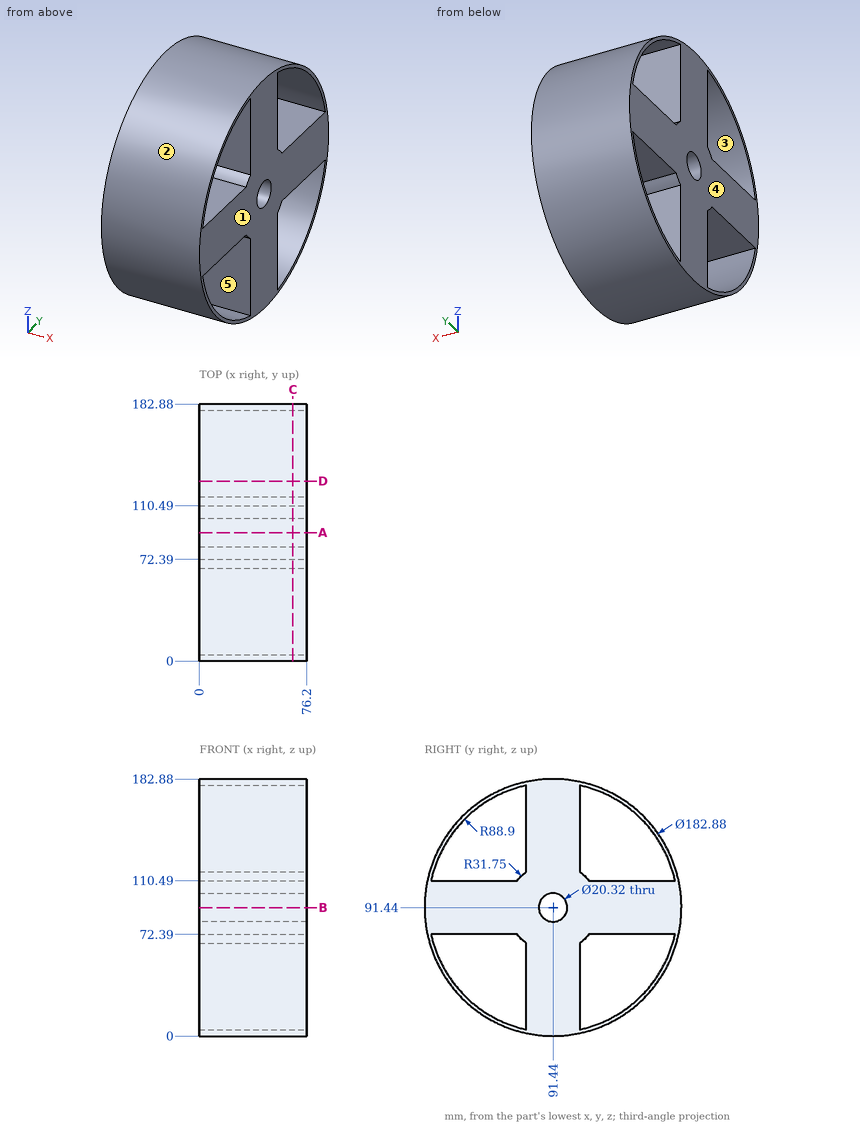
Drawing for the job (mm, zero at the part's lowest x, y, z). A direction names the side the tool comes from. Round coordinates to 2 decimals unless told otherwise and drop trailing zeros. Loops run counter-clockwise (first coordinate to the right, second up) from the corner with the lowest first, then second, coordinate; pieces in that order, holes last. Notation, with made-up numbers: (23, -28) -> (34, -28) arc R18 cw to (34, -18) -> close; hole circle Ø10 at (56.25, -13). An arc over 180 degrees is marked (long way). Answer in a Markdown table with one row per item.
Item 1: Mould opens along Z. For the marked faces 1, 2 and 3 say: +Z half, -Z half, draft (parallel to the pull), parting line (faces both ways), or undercut.
Answers below:
| item | result |
|---|---|
| face 1 | draft |
| face 2 | parting line |
| face 3 | undercut |
Item 2: Saw through at A-A (y = 91.44). Write the cut outline in (x, z), and give its area (3 significant figures).
Answers below:
| item | result |
|---|---|
| outline | (0, 0) -> (76.2, 0) -> (76.2, 81.28) -> (0, 81.28) -> close; (0, 101.6) -> (76.2, 101.6) -> (76.2, 182.88) -> (0, 182.88) -> close |
| area | 12,400 mm² |
Item 3: Saw through at D-D (y = 128). Write the cut outline in (x, z).
Answers below:
| item | result |
|---|---|
| outline | (0, 7.63) -> (76.2, 7.63) -> (76.2, 10.41) -> (0, 10.41) -> close; (0, 72.39) -> (76.2, 72.39) -> (76.2, 110.49) -> (0, 110.49) -> close; (0, 172.47) -> (76.2, 172.47) -> (76.2, 175.25) -> (0, 175.25) -> close |
Item 4: Which spindle directions (+Z, -Z, +X, -X, +Y, -Y) get a long thin tool onto all of the face, cutting with end or side? Do the marked faces 4 and 5. Say none if no direction does.
Answers below:
| item | result |
|---|---|
| face 4 | +Z, -Z, -X, +Y, -Y |
| face 5 | +X, -X |
Item 5: Saw through at C-C (x = 66.5). Write the cut outline in (y, z).
Answers below:
| item | result |
|---|---|
| outline | circle Ø182.88 at (91.44, 91.44); hole (4.61, 72.39) arc R88.9 ccw to (72.39, 4.61) -> (72.39, 66.04) arc R31.75 cw to (66.04, 72.39) -> close; hole (4.61, 110.49) -> (66.04, 110.49) arc R31.75 cw to (72.39, 116.84) -> (72.39, 178.27) arc R88.9 ccw to start; hole circle Ø20.32 at (91.44, 91.44); hole (110.49, 4.61) arc R88.9 ccw to (178.27, 72.39) -> (116.84, 72.39) arc R31.75 cw to (110.49, 66.04) -> close; hole (110.49, 116.84) arc R31.75 cw to (116.84, 110.49) -> (178.27, 110.49) arc R88.9 ccw to (110.49, 178.27) -> close |
Item 6: Drill centre lines: L1, parallel to Y at x = 52, z = 91.44; L2, parallel to Y at x = 58.5, z = 154.5; L3, parallel to Y at x = 67, z = 163.5. Where is each one in solid material? Low to high. Write a range as [from, to].
Answers below:
| item | result |
|---|---|
| L1 | y = [0, 81.28], [101.6, 182.88] |
| L2 | y = [25.22, 28.78], [72.39, 110.49], [154.1, 157.66] |
| L3 | y = [35.15, 39.38], [72.39, 110.49], [143.5, 147.73] |
Item 7: Pin check, flat tips, straight feed: pin 1 (4 mm diameter, centred on x = 19.5, y = 50.5, fed in from +Z); pin 2 (2 mm diameter, centred on x = 58.5, z = 135, fed in from -Y); pin 3 (2 mm diameter, centred on x = 11, y = 80, fed in from -Z). Stop position of each tip, or through.
Answers below:
| item | result |
|---|---|
| pin 1 | stops at z = 174.17 |
| pin 2 | stops at y = 10.51 |
| pin 3 | stops at z = 0.6 |
